Read the model definition and answer for the solid it produces. Units are mm, in the model's axes. Face numbers are marked on the shaded views. A direction names the side the tool comes from. Give positions to 0.01 mm unless a question says otherwise; leave off trailing zeros. Write each loop counter-clockwise with the first axis right and the second up, starting at its lowest first coordinate (ties: lowest second). Pieces come first, ordered by that corner, then holes. Notation, with made-up numbers: (-40, -14.5) -> (-9, -14.5) arc R19 cw to (-9, 0.5) -> close; hole circle Ø6 at (59, 33.5). An arc over 180 degrees is marked (long way). Write item = value, one per line.
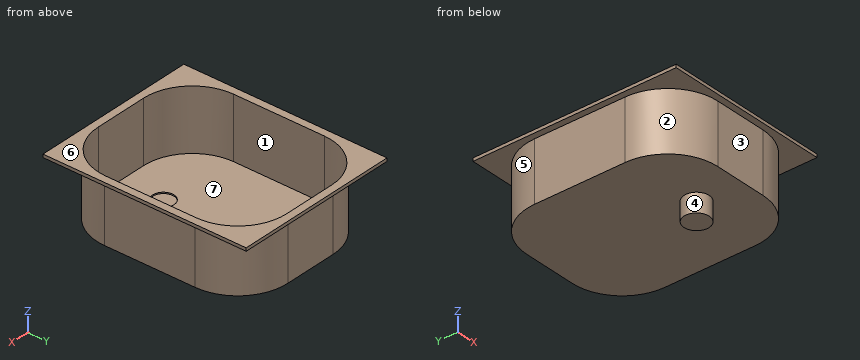
from build123d import *

# Parameters (mm, degrees)
F0_W     = 265
F0_H     = 325
F1_DEPTH = 5
F3_DEPTH = 95
F4_DEPTH = 25
F5_DEPTH = 98
F6_R     = 17
F7_DEPTH = 25
F6_R_2   = 20
F8_DEPTH = 30
F9_DEPTH = 5


with BuildPart() as f1:
    # F0 (on Top) → F1 (new body)
    with BuildSketch(Plane.XY):
        with Locations((132.5, 162.5)):
            Rectangle(F0_W, F0_H)
    extrude(amount=F1_DEPTH)

    # F2 (on face) → F3 (join)
    with BuildSketch(Plane(origin=(0, 0, 0), x_dir=(1, 0, 0), z_dir=(0, 0, -1))):
        with BuildLine():
            ThreePointArc((255, -90), (231.5685424949, -33.4314575051), (175, -10))
            Line((175, -10), (90, -10))
            ThreePointArc((90, -10), (33.4314575051, -33.4314575051), (10, -90))
            Line((10, -90), (10, -235))
            ThreePointArc((10, -235), (33.4314575051, -291.5685424949), (90, -315))
            Line((90, -315), (175, -315))
            ThreePointArc((175, -315), (231.5685424949, -291.5685424949), (255, -235))
            Line((255, -235), (255, -90))
        make_face()
        with BuildLine():
            ThreePointArc((175, -12), (230.1543289326, -34.8456710674), (253, -90))
            Line((253, -90), (253, -235))
            ThreePointArc((253, -235), (230.1543289326, -290.1543289326), (175, -313))
            Line((175, -313), (90, -313))
            ThreePointArc((90, -313), (34.8456710674, -290.1543289326), (12, -235))
            Line((12, -235), (12, -90))
            ThreePointArc((12, -90), (34.8456710674, -34.8456710674), (90, -12))
            Line((90, -12), (175, -12))
        make_face(mode=Mode.SUBTRACT)
        with BuildLine():
            Line((253, -235), (253, -90))
            ThreePointArc((253, -90), (230.1543289326, -34.8456710674), (175, -12))
            Line((175, -12), (90, -12))
            ThreePointArc((90, -12), (34.8456710674, -34.8456710674), (12, -90))
            Line((12, -90), (12, -235))
            ThreePointArc((12, -235), (34.8456710674, -290.1543289326), (90, -313))
            Line((90, -313), (175, -313))
            ThreePointArc((175, -313), (230.1543289326, -290.1543289326), (253, -235))
        make_face()
    extrude(amount=F3_DEPTH)

    # F2 (on face) → F4 (cut)
    with BuildSketch(Plane(origin=(0, 0, 0), x_dir=(1, 0, 0), z_dir=(0, 0, -1))):
        with BuildLine():
            ThreePointArc((255, -90), (231.5685424949, -33.4314575051), (175, -10))
            Line((175, -10), (90, -10))
            ThreePointArc((90, -10), (33.4314575051, -33.4314575051), (10, -90))
            Line((10, -90), (10, -235))
            ThreePointArc((10, -235), (33.4314575051, -291.5685424949), (90, -315))
            Line((90, -315), (175, -315))
            ThreePointArc((175, -315), (231.5685424949, -291.5685424949), (255, -235))
            Line((255, -235), (255, -90))
        make_face()
        with BuildLine():
            ThreePointArc((175, -12), (230.1543289326, -34.8456710674), (253, -90))
            Line((253, -90), (253, -235))
            ThreePointArc((253, -235), (230.1543289326, -290.1543289326), (175, -313))
            Line((175, -313), (90, -313))
            ThreePointArc((90, -313), (34.8456710674, -290.1543289326), (12, -235))
            Line((12, -235), (12, -90))
            ThreePointArc((12, -90), (34.8456710674, -34.8456710674), (90, -12))
            Line((90, -12), (175, -12))
        make_face(mode=Mode.SUBTRACT)
    extrude(amount=-F4_DEPTH, mode=Mode.SUBTRACT)

    # F5 (cut): a face of the model
    f5_faces = [f1.faces().sort_by_distance(p)[0] for p in [
        (132.5, 162.5, 5),
    ]]
    extrude(f5_faces, amount=-F5_DEPTH, mode=Mode.SUBTRACT)

    # F6 (on face) → F7 (cut)
    with BuildSketch(Plane(origin=(0, 0, -95), x_dir=(1, 0, 0), z_dir=(0, 0, -1))):
        with Locations((132.5, -80)):
            Circle(F6_R)
    extrude(amount=-F7_DEPTH, mode=Mode.SUBTRACT)

    # F6 (on face) → F8 (join)
    with BuildSketch(Plane(origin=(0, 0, -95), x_dir=(1, 0, 0), z_dir=(0, 0, -1))):
        with Locations((132.5, -80)):
            Circle(F6_R_2)
        with Locations((132.5, -80)):
            Circle(F6_R, mode=Mode.SUBTRACT)
        with Locations((132.5, -80)):
            Circle(F6_R)
    extrude(amount=F8_DEPTH)

    # F9 (add): a face of the model
    f9_faces = [f1.faces().sort_by_distance(p)[0] for p in [
        (231.2919109711, 33.7080890289, 0),
    ]]
    extrude(f9_faces, amount=F9_DEPTH)


solid = f1.part
(1) A tool of negligible diameter and unlimited length cuts with its end or side. For the marked faces 1, 2, 3 and 4, from which of +Z, -Z, +X, -X, +Y, -Y can it reach the whole face along a straight path? Write none if from no direction.
Checks:
face_1 = +Z
face_2 = -Z, -X, -Y
face_3 = -Z, +X, -X, -Y
face_4 = -Z
(2) Consider L1, parallel to Y at x = 162, z = -81; L2, parallel to X at y = 220.5, z = -49; L3, parallel to Y at x = 132.5, z = -94.1. Determine where each line is inside the solid, lowest interval first.
Checks:
L1 = 10 to 12, 313 to 315
L2 = 10 to 12, 253 to 255
L3 = 10 to 63, 97 to 315
(3) The part is cut by section D-D on z = -112. Determine the outline of the cut face in (x, y).
Checks:
outline = circle Ø40 at (132.5, 80)
(4) The part is cut by section B-B on y = 146. Determine the outline of the cut face in (x, z).
Checks:
outline = (0, 0) -> (10, 0) -> (10, -95) -> (255, -95) -> (255, 0) -> (265, 0) -> (265, 5) -> (253, 5) -> (253, -93) -> (12, -93) -> (12, 5) -> (0, 5) -> close
(5) The part is cut by section C-C on z = -31. Determine the outline of the cut face in (x, y), plus the area to 3 significant figures.
Checks:
outline = (10, 90) arc R80 ccw to (90, 10) -> (175, 10) arc R80 ccw to (255, 90) -> (255, 235) arc R80 ccw to (175, 315) -> (90, 315) arc R80 ccw to (10, 235) -> close; hole (12, 90) arc R78 ccw to (90, 12) -> (175, 12) arc R78 ccw to (253, 90) -> (253, 235) arc R78 ccw to (175, 313) -> (90, 313) arc R78 ccw to (12, 235) -> close
area = 1,910 mm²
(6) The part is cut by section A-A on x = 132.5. Determine the outline of the cut face in (y, z).
Checks:
outline = (0, 0) -> (10, 0) -> (10, -95) -> (60, -95) -> (60, -125) -> (100, -125) -> (100, -95) -> (315, -95) -> (315, 0) -> (325, 0) -> (325, 5) -> (313, 5) -> (313, -93) -> (97, -93) -> (97, -95) -> (63, -95) -> (63, -93) -> (12, -93) -> (12, 5) -> (0, 5) -> close
(7) Given P1, Ø4, axis at x = 60.5, z = -16.5, coming from the -Y side; P2, Ø1.5, axis at x = 133, y = 155, coming from the -Z side; P3, Ø12, axis at y = 188, z = -47.5, coming from the +X side, each flat-ended and moving along its own axis, determine where each tip first touches the part or whether it passes through.
Checks:
P1 = 14.88
P2 = -95
P3 = 255
(8) For a pull along Y with two mould halves and no side action, classify the marked faces 5, 6 and 7 as released by +Y, released by -Y, zero draft, split by the parting line, or undercut.
Checks:
face_5 = released by +Y
face_6 = zero draft
face_7 = undercut
